```python
from build123d import *

# Parameters (mm, degrees)
SKETCH1_R           = 12.319
BOSS_EXTRUDE1_DEPTH = 46.99
SKETCH2_R           = 5.842
BOSS_EXTRUDE2_DEPTH = 2.286
SKETCH3_R           = 1.905
BOSS_EXTRUDE3_DEPTH = 10.16
SKETCH4_W           = 43.053
SKETCH4_H           = 0.0254
FILLET1_R           = 1.27
SKETCH5_R           = 3.048
BOSS_EXTRUDE4_DEPTH = 3.81
FILLET2_R           = 2.54
SKETCH6_R           = 1.016
CUT_EXTRUDE1_DEPTH  = 6.35
SKETCH7_W           = 2.991253898
SKETCH7_H           = 0.508
CUT_EXTRUDE2_DEPTH  = 10.16


with BuildPart() as part:
    # Sketch1 → Boss-Extrude1 (new body)
    with BuildSketch(Plane.XY):
        Circle(SKETCH1_R)
    extrude(amount=-BOSS_EXTRUDE1_DEPTH)

    # Sketch2 → Boss-Extrude2 (add)
    with BuildSketch(Plane.XY):
        Circle(SKETCH2_R)
    extrude(amount=BOSS_EXTRUDE2_DEPTH)

    # Sketch3 → Boss-Extrude3 (add)
    with BuildSketch(Plane.XY.offset(2.286)):
        Circle(SKETCH3_R)
    extrude(amount=BOSS_EXTRUDE3_DEPTH)

    # Sketch4 → Cut-Revolve1 (revolve, cut)
    with BuildSketch(Plane(origin=(0, 0, 0), x_dir=(0, 0, -1), z_dir=(1, 0, 0))):
        with Locations((25.4635, 12.3063)):
            Rectangle(SKETCH4_W, SKETCH4_H)
    revolve(axis=Axis((0, 0, -46.99), (0, 0, 1)), mode=Mode.SUBTRACT)

    # Fillet1
    fillet1_edges = [part.edges().sort_by_distance(p)[0] for p in [
        (0, -12.2936, -46.99),
    ]]
    fillet(fillet1_edges, radius=FILLET1_R)

    # Sketch5 → Boss-Extrude4 (add)
    with BuildSketch(Plane(origin=(0, 0, -46.99), x_dir=(-1, 0, 0), z_dir=(0, 0, -1))):
        with Locations((0, 7.62)):
            Circle(SKETCH5_R)
    extrude(amount=BOSS_EXTRUDE4_DEPTH)

    # Fillet2
    fillet2_edges = [part.edges().sort_by_distance(p)[0] for p in [
        (3.048, 7.62, -50.8),
    ]]
    fillet(fillet2_edges, radius=FILLET2_R)

    # Sketch6 → Cut-Extrude1 (cut)
    with BuildSketch(Plane.XY):
        with Locations((0, 9.398)):
            Circle(SKETCH6_R)
    cut_extrude1 = extrude(amount=-CUT_EXTRUDE1_DEPTH, mode=Mode.SUBTRACT)

    # Mirror1: Cut-Extrude1 across plane
    add(cut_extrude1.mirror(Plane.ZX), mode=Mode.SUBTRACT)

    # Sketch7 → Cut-Extrude2 (cut)
    with BuildSketch(Plane.XY.offset(12.446)):
        with Locations((0, 1.672065055)):
            Rectangle(SKETCH7_W, SKETCH7_H)
    extrude(amount=-CUT_EXTRUDE2_DEPTH, mode=Mode.SUBTRACT)


solid = part.part
```
Source: CAD feature listing. Evaluate the final solid. Frame: model axes, mm. A direction names the side the tool comes from. Coordinates: 2 decimals unless noted, no trailing zeros. Order: outer loops, then holes, each group sorted by start corner. A loop starts at its lowest first (then second) coordinate and runs counter-clockwise, first axis right, second up. Notation, with made-up numbers: M 43.25,0 L 55.25,0 A20 cw 55.25,27 Z; hole C 54.5,13 d1. An arc over 180 degrees is marked long. Write each question's results on one line, items separated by ' | '. Start each with the question number.
1) Draft query along Y for faces 1 (the face through (0, 9, -6.35)), 2 (the face through (0, 1.418, 7)), 3 (the face through (-1.266, -5.703, 1.127)). Return one class per face: released by +Y, released by -Y, zero draft, split by the parting line, or undercut.
2) Access query for faces 4 (the face through (0.4, 10.64, -47.62)), 5 (the face through (0, -3, 2.286)). Directions: +Z, -Z, +X, -X, +Y, -Y. A direction counts if a zero-diameter tool reaches every point of the face in a straight line with its end or side. Return the directions, or none.
3) Section query C-C (z = -2). Return the cut outline in (x, y), plus the area to 3 significant figures.
4) Contact query for flat-ended pins moving along their axis: pin 1 Ø0.6 at (x, y) = (0.5, -10) entering from +Z; pin 2 Ø10 at (y, z) = (-1.5, -41.5) entering from -X; pin 3 Ø1.5 at (x, y) = (6.5, -4.5) entering from -Z. Output: stop coordinate, or through.
5) Section query B-B (z = -26). Return the cut outline in (x, y), plus the area to 3 significant figures.
6) Section query A-A (y = 0). Return the cut outline in (x, z) (3 decimals).
7) Line query: line 1 (Y direction, x = 0, z = -5); line 2 (Z direction, x = 1.5, y = 3.5); line 3 (Z direction, x = 5.25, y = -6). Output: solid intervals per line, ascending. Write a range as from..to.
Answers:
1) face 1: undercut | face 2: released by +Y | face 3: split by the parting line
2) face 4: -Z | face 5: +Z
3) outline: C 0,0 d24.64; hole C 0,-9.4 d2.03; hole C 0,9.4 d2.03 | area: 470 mm^2
4) pin 1: stops at z = 0 | pin 2: stops at x = -12.29 | pin 3: stops at z = -46.99
5) outline: C 0,0 d24.59 | area: 475 mm^2
6) outline: M -12.319,-3.937 L -12.294,-3.937 L -12.294,-45.72 A1.27 ccw -11.024,-46.99 L 11.024,-46.99 A1.27 ccw 12.294,-45.72 L 12.294,-3.937 L 12.319,-3.937 L 12.319,0 L 5.842,0 L 5.842,2.286 L 1.905,2.286 L 1.905,12.446 L -1.905,12.446 L -1.905,2.286 L -5.842,2.286 L -5.842,0 L -12.319,0 Z
7) line 1: y = -12.29..-10.41, -8.38..8.38, 10.41..12.29 | line 2: z = -46.99..2.29 | line 3: z = -46.99..0
